Geometry: see drawing. Coordinates: mm, zero at the bounding-box minimum. A direction names the side the tool comes from. Give positions to 0.01 mm unless a question says otherwise; leave off trailing zeros. Write each loop counter-clockwise with the first axis right and the second up, starting at its lowest first coordinate (ties: lowest second). Pieces come first, ordered by that corner, then holes. Notation, with made-up numbers: (63.25, 66) -> (77.25, 66) arc R7 cw to (77.25, 71) -> close; hole circle Ø3 at (-33.75, 61.5). An arc over 180 degrees is marked (long way). Use CSV: the item, a comma, the result in double quotes. Start each with the question number.
1) Set-up query: the marked faces 1 and 2. Return all of +Z, -Z, +X, -X, +Y, -Y with unobstructed straight access to the full face (end or side cutting, diameter ignored); none if empty.
2) Section A-A (y = 13.75). Output: boundary loops of the cut face in (x, z).
3) Section C-C (z = 11). Output: boundary loops of the cut face in (x, y), plus the area to 3 significant figures.
4) Section B-B (x = 46.5). Output: boundary loops of the cut face in (y, z).
5) Contact query for flat-ended pins moving along their axis: P1, Ø3, axis at x = 6.5, z = 14, coming from the -Y side; P2, Ø5, axis at x = 6.5, z = 13, coming from the +Y side; P3, Ø0.5, axis at x = 17.5, z = 5, coming from the +Y side. Output: stop coordinate, or through.
6) Material intervals for line 1 (Z direction, x = 6.5, y = 12); line 2 (Z direction, x = 19, y = 8.75); line 3 (Y direction, x = 8, z = 11), sorted ascending. Write a range as [from, to].
7) Section D-D (y = 5.5). Output: boundary loops of the cut face in (x, z).
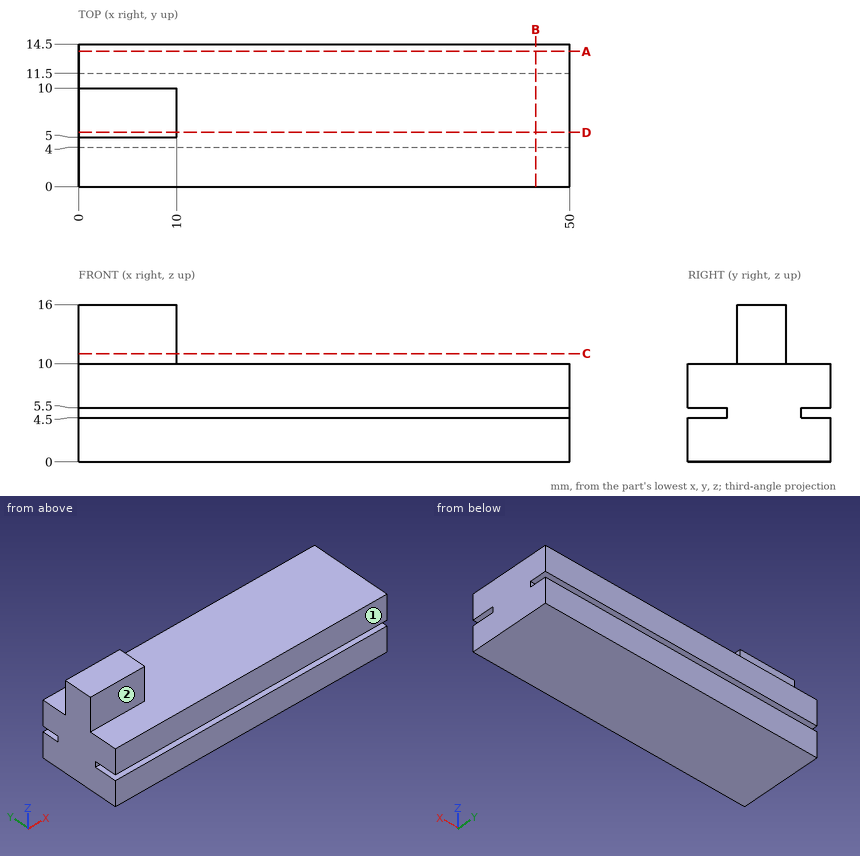
Answers follow:
1,face 1,"+Z, -Z, +X, -X, -Y"
1,face 2,"+Z, +X, -X, -Y"
2,outline,"(0, 0) -> (50, 0) -> (50, 4.5) -> (0, 4.5) -> close; (0, 5.5) -> (50, 5.5) -> (50, 10) -> (0, 10) -> close"
3,outline,"(0, 5) -> (10, 5) -> (10, 10) -> (0, 10) -> close"
3,area,"50.0 mm^2"
4,outline,"(0, 0) -> (14.5, 0) -> (14.5, 4.5) -> (11.5, 4.5) -> (11.5, 5.5) -> (14.5, 5.5) -> (14.5, 10) -> (0, 10) -> (0, 5.5) -> (4, 5.5) -> (4, 4.5) -> (0, 4.5) -> close"
5,P1,"stops at y = 5"
5,P2,"stops at y = 10"
5,P3,"stops at y = 11.5"
6,line 1,"z = [0, 4.5], [5.5, 10]"
6,line 2,"z = [0, 10]"
6,line 3,"y = [5, 10]"
7,outline,"(0, 0) -> (50, 0) -> (50, 10) -> (10, 10) -> (10, 16) -> (0, 16) -> close"
